Read the model definition and answer for the solid it produces. Units are mm, in the model's axes. A direction names the side the tool comes from. Give positions to 0.01 mm unless a question says otherwise; leave off trailing zeros. Order: outer loops, then holes, each group sorted by start corner. A loop starts at its lowest first (then second) coordinate and runs counter-clockwise, first axis right, second up.
```python
from build123d import *

# Parameters (mm, degrees)
SKETCH_1_W          = 10
SKETCH_1_H          = 10
EXTRUDE_1_DEPTH     = 1
SKETCH_2_W          = 6
SKETCH_2_H          = 4.5
EXTRUDE_2_DEPTH     = 0.2
SKETCH_3_W          = 30
SKETCH_3_H          = 30
EXTRUDE_3_DEPTH     = 1.5
SKETCH_4_R          = 1
CUT_EXTRUDE_2_DEPTH = 22.266170318


with BuildPart() as part:
    # Sketch 1 → Extrude 1 (new body)
    with BuildSketch(Plane(origin=(0, 0, 0), x_dir=(1, 0, 0), z_dir=(0, 1, 0))):
        Rectangle(SKETCH_1_W, SKETCH_1_H)
    extrude(amount=EXTRUDE_1_DEPTH)

    # Sketch 2 → Extrude 2 (add)
    with BuildSketch(Plane(origin=(0, 1, 0), x_dir=(1, 0, 0), z_dir=(0, 1, 0))):
        Rectangle(SKETCH_2_W, SKETCH_2_H)
    extrude(amount=EXTRUDE_2_DEPTH)

    # Sketch 3 → Extrude 3 (add)
    with BuildSketch(Plane.XZ):
        Rectangle(SKETCH_3_W, SKETCH_3_H)
    extrude(amount=EXTRUDE_3_DEPTH)

    # Sketch 4 → Cut-Extrude 2 (cut, through all)
    with BuildSketch(Plane(origin=(0, 0, 0), x_dir=(1, 0, 0), z_dir=(0, 1, 0))):
        with Locations(Location((9, 0, 0), (0, 0, 270))):
            Circle(SKETCH_4_R)
        with Locations(Location((-9, 0, 0), (0, 0, 270))):
            Circle(SKETCH_4_R)
    extrude(amount=-CUT_EXTRUDE_2_DEPTH, mode=Mode.SUBTRACT)


solid = part.part
```
1) Consider L1, parallel to X at y = -0.5, z = 0; L2, parallel to Y at x = -3.75, z = -3.5; L3, parallel to Y at x = -1.25, z = -13.5. Determine where each line is inside the solid, lowest interval first.
Final values:
L1: x = -15 to -10, -8 to 8, 10 to 15
L2: y = -1.5 to 1
L3: y = -1.5 to 0
2) A tool of negligible diameter and unlimited length cuts with its end or side. For faces 5 (the face through (-5, 0.5, 0.1)), 6 (the face through (-0.1, 0.5, 5)), 7 (the face through (-0.1, 0.5, -5)), from which of +Z, -Z, +X, -X, +Y, -Y can it reach the whole face along a straight path? Write none if from no direction.
Final values:
face 5: +Z, -Z, -X, +Y
face 6: +Z, +X, -X, +Y
face 7: -Z, +X, -X, +Y
3) The part is cut by section B-B on x = 9. Determine the outline of the cut face in (y, z), and give its area (3 significant figures).
Final values:
outline: (-1.5, -15) - (0, -15) - (0, -1) - (-1.5, -1) - close; (-1.5, 1) - (0, 1) - (0, 15) - (-1.5, 15) - close
area: 42.0 mm2
4) For a pull along X with two mould halves and no side action, classify faces 1 (the face through (-8, -1, 0)), 2 (the face through (5, 0.5, 0.1)), 3 (the face through (0, -1, 15)), 4 (the face through (10, -1, 0)) as released by +X, released by -X, zero draft, split by the parting line, or undercut.
Final values:
face 1: undercut
face 2: released by +X
face 3: zero draft
face 4: undercut
5) The part is cut by section C-C on x = -4. Determine the outline of the cut face in (y, z).
Final values:
outline: (-1.5, -15) - (0, -15) - (0, -5) - (1, -5) - (1, 5) - (0, 5) - (0, 15) - (-1.5, 15) - close
6) The part is cut by section D-D on z = 7.75. Determine the outline of the cut face in (x, y), and give its area (3 significant figures).
Final values:
outline: (-15, -1.5) - (15, -1.5) - (15, 0) - (-15, 0) - close
area: 45.0 mm2
7) The part is cut by section A-A on z = 0. Determine the outline of the cut face in (x, y).
Final values:
outline: (-15, -1.5) - (-10, -1.5) - (-10, 0) - (-15, 0) - close; (-8, -1.5) - (8, -1.5) - (8, 0) - (5, 0) - (5, 1) - (3, 1) - (3, 1.2) - (-3, 1.2) - (-3, 1) - (-5, 1) - (-5, 0) - (-8, 0) - close; (10, -1.5) - (15, -1.5) - (15, 0) - (10, 0) - close
8) Given pin 1 (2.5 mm diameter, centred on x = -9, z = 0, fed in from -Y); pin 2 (0.8 mm diameter, centred on y = 0.5, z = 1, fed in from +X); pin 3 (0.8 mm diameter, centred on y = 0.5, z = 2.5, fed in from -X); pin 4 (0.5 mm diameter, centred on x = -2, y = 0.5, fed in from -Z), each flat-ended and moving along its own axis, determine where each tip first touches the part or whether it passes through.
Final values:
pin 1: stops at y = -1.5
pin 2: stops at x = 5
pin 3: stops at x = -5
pin 4: stops at z = -5
